Read the model definition and answer for the solid it produces. Units are mm, in the model's axes. A direction names the side the tool comes from. Round coordinates to 2 decimals unless told otherwise and drop trailing zeros. Loops run counter-clockwise (first coordinate to the right, second up) from the corner with the lowest first, then second, coordinate; pieces in that order, holes last. Notation, with made-up numbers: (-33, -37) - (5, -37) arc R11 cw to (5, -20) - close; hole circle Ø4 at (10.25, -22). An arc over 180 degrees is marked (long way). Use CSV: the item, a comma, the result in double quotes. Start each with the question number.
1. Find section D-D (x = 0). Give the vertices of the cut face in (y, z), and give its area (3 significant figures).
2. Consider line 1 along Y through (x, z) = (-20, 1.7); line 2 along X through (y, z) = (23, 1.5); line 3 along X through (y, z) = (28, 0.6). Determine where each line is inside the solid, lowest interval first.
3. Find section C-C (z = 0.9). State how many separate pieces and enclosed holes the cut face has, and give its area (3 significant figures).
4. Find section A-A (x = 44). Give the vertices of the cut face in (y, z).
5. A tool of negligible diameter and unlimited length cuts with its end or side. For faces 3 (the cylindrical face through (67.664, 10.503, 1.521)), 4 (the flat face through (-1, 6, 0)), from which of +Z, -Z, +X, -X, +Y, -Y can it reach the whole face along a straight path? Write none if from no direction.
6. Find section B-B (x = 76). Give the vertices of the cut face in (y, z).
7. Determine the mould class of faces 1 (the flat face through (-1, 6, 3)), 2 (the cylindrical face through (67.136, 46.997, 1.521)) for opening direction Y: +Y half, -Y half, draft (parallel to the pull), parting line (faces both ways), or undercut.
8. Given pin 1 Ø0.9 at (y, z) = (26.5, 1) entering from +X; pin 2 Ø0.9 at (x, z) = (98, 1) entering from -Y; pin 3 Ø1.5 at (y, z) = (-26.5, 1) entering from +X, each flat-ended and moving along its own axis, determine where each tip first touches the part or whether it passes through.
from build123d import *

# Parameters (mm, degrees)
BOSS_EXTRUDE1_DEPTH = 3
SKETCH2_W           = 15
SKETCH2_H           = 3
CUT_EXTRUDE1_DEPTH  = 10


with BuildPart() as part:
    # Sketch1 → Boss-Extrude1 (new body)
    with BuildSketch(Plane.XY):
        Polygon((-97, -12.5), (-97, -25.5), (-83.5, -25.5), (-83.5, -28.5), (-68.5, -28.5), (-68.5, -25.5), (-52.5, -25.5), (-52.5, -28.5), (-37.5, -28.5), (-37.5, -25.5), (-22.5, -25.5), (-22.5, -28.5), (-7.5, -28.5), (-7.5, -25.5), (0, -25.5), (7.5, -25.5), (7.5, -28.5), (22.5, -28.5), (22.5, -25.5), (30, -25.5), (37.5, -25.5), (37.5, -28.5), (52.5, -28.5), (52.5, -25.5), (60, -25.5), (67.5, -25.5), (67.5, -28.5), (82.5, -28.5), (82.5, -25.5), (97, -25.5), (97, -12.5), (100, -12.5), (100, -2.5), (97, -2.5), (97, 7.5), (100, 7.5), (100, 17.5), (97, 17.5), (97, 27.5), (100, 27.5), (100, 37.5), (97, 37.5), (97, 47.5), (100, 47.5), (100, 57.5), (97, 57.5), (-97, 57.5), (-100, 57.5), (-100, 47.5), (-97, 47.5), (-97, 37.5), (-100, 37.5), (-100, 27.5), (-97, 27.5), (-97, 17.5), (-100, 17.5), (-100, 7.5), (-97, 7.5), (-97, -2.5), (-100, -2.5), (-100, -12.5), align=None)
    extrude(amount=BOSS_EXTRUDE1_DEPTH)

    # Sketch2 → Cut-Extrude1 (cut)
    with BuildSketch(Plane.XY.offset(3)):
        with BuildLine():
            Line((55.4, 22.5), (55.4, 35))
            ThreePointArc((55.4, 35), (67.4, 47), (79.4, 35))
            Line((79.4, 35), (79.4, 22.5))
            ThreePointArc((79.4, 22.5), (67.4, 10.5), (55.4, 22.5))
        make_face()
        with Locations((15, 7.5)):
            Rectangle(SKETCH2_W, SKETCH2_H)
        with Locations((45, 7.5)):
            Rectangle(SKETCH2_W, SKETCH2_H)
        with Locations((75, 7.5)):
            Rectangle(SKETCH2_W, SKETCH2_H)
        with Locations((-75, 7.5)):
            Rectangle(SKETCH2_W, SKETCH2_H)
        with Locations((-45, 7.5)):
            Rectangle(SKETCH2_W, SKETCH2_H)
        with Locations((-15, 7.5)):
            Rectangle(SKETCH2_W, SKETCH2_H)
        with BuildLine():
            Line((-7.5, 11), (-7.5, 16.5))
            ThreePointArc((-7.5, 16.5), (0, 24), (7.5, 16.5))
            Line((7.5, 16.5), (7.5, 11))
            Line((7.5, 11), (5.5, 9))
            Line((5.5, 9), (-5.5, 9))
            Line((-5.5, 9), (-7.5, 11))
        make_face()
    extrude(amount=-CUT_EXTRUDE1_DEPTH, mode=Mode.SUBTRACT)


solid = part.part
Filled sheet:
1,outline,"(-25.5, 0) - (9, 0) - (9, 3) - (-25.5, 3) - close; (24, 0) - (57.5, 0) - (57.5, 3) - (24, 3) - close"
1,area,"204 mm²"
2,line 1,"y = -28.5 to 6, 9 to 57.5"
2,line 2,"x = -97 to -3.74, 3.74 to 55.4, 79.4 to 97"
2,line 3,"x = -100 to 55.4, 79.4 to 100"
3,separate pieces,"1"
3,enclosed holes,"8"
3,area,"15,400 mm²"
4,outline,"(-28.5, 0) - (6, 0) - (6, 3) - (-28.5, 3) - close; (9, 0) - (57.5, 0) - (57.5, 3) - (9, 3) - close"
5,face 3,"+Z, -Z"
5,face 4,"-Z, +X, -X, +Y, -Y"
6,outline,"(-28.5, 0) - (6, 0) - (6, 3) - (-28.5, 3) - close; (9, 0) - (14.13, 0) - (14.13, 3) - (9, 3) - close; (43.37, 0) - (57.5, 0) - (57.5, 3) - (43.37, 3) - close"
7,face 1,"draft"
7,face 2,"undercut"
8,pin 1,"stops at x = 97"
8,pin 2,"stops at y = -12.5"
8,pin 3,"stops at x = 82.5"
